from build123d import *

# Parameters (mm, degrees)
F0_W     = 30
F0_H     = 10
F0_R     = 2.5
F1_DEPTH = 25
F2_R     = 4
F3_DEPTH = 5
F4_R     = 5
F5_DEPTH = 25


with BuildPart() as f1:
    # F0 (on Top) → F1 (new body)
    with BuildSketch(Plane.XY):
        with Locations((15, 5)):
            Rectangle(F0_W, F0_H)
        with Locations((5, 5)):
            Circle(F0_R, mode=Mode.SUBTRACT)
        with Locations((25, 5)):
            Circle(F0_R, mode=Mode.SUBTRACT)
    extrude(amount=F1_DEPTH)

    # F2 (on face) → F3 (cut)
    with BuildSketch(Plane.XY.offset(25)):
        with Locations((5, 5)):
            Circle(F2_R)
        with Locations((25, 5)):
            Circle(F2_R)
    extrude(amount=-F3_DEPTH, mode=Mode.SUBTRACT)

    # F4 (on face) → F5 (cut)
    with BuildSketch(Plane.XZ):
        with Locations((15, 15)):
            Circle(F4_R)
    extrude(amount=-F5_DEPTH, mode=Mode.SUBTRACT)


solid = f1.part
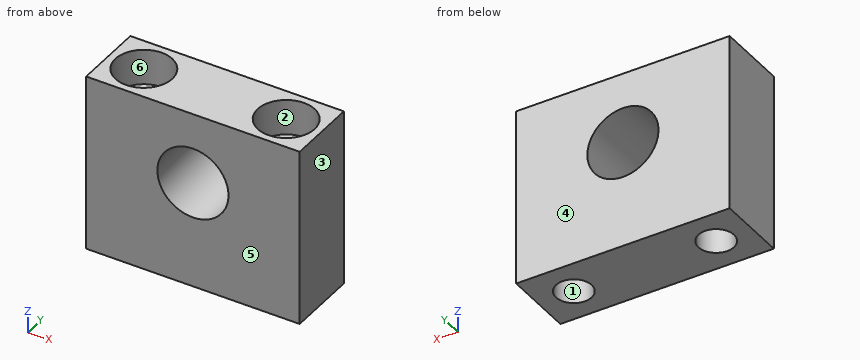
Can you work these out from the model? Positions are in its coordinate system, mm. Face numbers are marked on the shaded views. A direction names the side the tool comes from. Give positions to 0.01 mm unless a question says otherwise; leave off trailing zeros. Write each loop counter-clockwise with the first axis right and the second up, starting at its lowest first coordinate (ties: lowest second). Pieces come first, ordered by that corner, then holes. Notation, with made-up numbers: M 15.25,60 L 56.25,60 A11 cw 56.25,66 Z; hole C -21.75,68.5 d1. An arc over 180 degrees is marked long. Answer in a Markdown table with one row per item. Add a question column.
Item 1: Please list where these lines run through material, in increasing order: L1, parallel to X at y = 5, z = 6.5; L2, parallel to Y at x = 25, z = 12.25; L3, parallel to Y at x = 5, z = 22.25.
Item 2: Imagine slicing it at D-D, the plane z = 4.75. Write out the boundary of the cut face in (x, y).
Item 3: We'd pull the mould along Y, two halves only. Please class the marked faces 1, 2, 3 and 4: released by +Y, released by -Y, zero draft, split by the parting line, or undercut.
Item 4: Imagine slicing it at A-A, the plane z = 15. Write out the boundary of the cut face in (x, y).
Item 5: On a 3-axis mill with a long thin cutter (end or side, diameter ignored), from which of +Z, -Z, +X, -X, +Y, -Y can I reach the whole of each face in a straight line? I mean the marked faces 5 and 6. Say none if no direction works.
Item 6: Imagine slicing it at B-B, the plane y = 5. Write out the boundary of the cut face in (x, z).
Item 7: Imagine slicing it at C-C, the plane x = 15. Write out the boundary of the cut face in (y, z).
Evaluation:
| question | item | result |
|---|---|---|
| 1 | L1 | x = 0 to 2.5, 7.5 to 22.5, 27.5 to 30 |
| 1 | L2 | y = 0 to 2.5, 7.5 to 10 |
| 1 | L3 | y = 0 to 1, 9 to 10 |
| 2 | outline | M 0,0 L 30,0 L 30,10 L 0,10 Z; hole C 5,5 d5; hole C 25,5 d5 |
| 3 | face 1 | undercut |
| 3 | face 2 | undercut |
| 3 | face 3 | zero draft |
| 3 | face 4 | released by +Y |
| 4 | outline | M 0,0 L 10,0 L 10,10 L 0,10 Z; M 20,0 L 30,0 L 30,10 L 20,10 Z; hole C 5,5 d5; hole C 25,5 d5 |
| 5 | face 5 | +Z, -Z, +X, -X, -Y |
| 5 | face 6 | +Z |
| 6 | outline | M 0,0 L 2.5,0 L 2.5,20 L 1,20 L 1,25 L 0,25 Z; M 7.5,0 L 22.5,0 L 22.5,20 L 21,20 L 21,25 L 9,25 L 9,20 L 7.5,20 Z; M 27.5,0 L 30,0 L 30,25 L 29,25 L 29,20 L 27.5,20 Z; hole C 15,15 d10 |
| 7 | outline | M 0,0 L 10,0 L 10,10 L 0,10 Z; M 0,20 L 10,20 L 10,25 L 0,25 Z |
